Design review of the part built by this model. Coordinates are the model's own, in mm. A direction names the side the tool comes from. Give positions to 0.01 mm unless a question says otherwise; leave off trailing zeros. Loops run counter-clockwise (first coordinate to the right, second up) from the corner with the lowest first, then second, coordinate; pieces in that order, holes last. Notation, with made-up numbers: (40.5, 68) - (82.5, 68) arc R27 cw to (82.5, 89) - close; hole circle Ø8 at (84.5, -14.75). An arc over 180 degrees is marked (long way). One line per item, written item: value. Start each with the question number.
```python
from build123d import *

# Parameters (mm, degrees)
F0_R     = 6.2
F0_R_2   = 5
F1_DEPTH = 10
F0_R_3   = 3.8
F2_DEPTH = 20
F3_SIZE  = 0.5


with BuildPart() as f1:
    # F0 (on Top) → F1 (new body)
    with BuildSketch(Plane.XY):
        Circle(F0_R)
        Circle(F0_R_2, mode=Mode.SUBTRACT)
    extrude(amount=F1_DEPTH)

    # F0 (on Top) → F2 (join)
    with BuildSketch(Plane.XY):
        Circle(F0_R_2)
        Circle(F0_R_3, mode=Mode.SUBTRACT)
    extrude(amount=F2_DEPTH)

    # F3
    f3_edges = [f1.edges().sort_by_distance(p)[0] for p in [
        (-5, 0, 20),
    ]]
    chamfer(f3_edges, length=F3_SIZE)


solid = f1.part
```
(1) To check wall thickness, follow L1, parallel to Y at x = 0, z = 8; L2, parallel to Z at x = -2.5, y = 5; L3, parallel to Y at x = -1.75, z = 3. State the ranges of each line that lie inside material, in increasing order. Write a range as from..to.
(2) Take a section at C-C on z = 2. State the section outline as (x, y) points, and give its area (3 significant figures).
(3) Take a section at D-D on z = 12.5. State the section outline as (x, y) points.
(4) Machinability: for faces 1 (the cylindrical face through (-1.08, -4.88, 14.68)), 2 (the flat face through (-4, -1, 20)), which of the approach directions +Z, -Z, +X, -X, +Y, -Y give a long, thin tool a straight path to every point of the face, cutting with its end or side? Answer none if there is none.
(5) For pin 1 Ø1.5 at (x, y) = (-4.5, 3.5) entering from +Z; pin 2 Ø1.5 at (x, z) = (5, 5) entering from +Y; pin 3 Ø1.5 at (y, z) = (4, 12.5) entering from -X, all flat-tipped, find the tip position at first contact; note any pin that passes through.
(6) Take a section at A-A on y = 0. State the section outline as (x, z) points.
(7) Draft analysis for pull direction X (two halves, no side actions). For faces 3 (the cylindrical face through (2.86, -5.5, 4.93)), 4 (the flat face through (3, 3, 0)), 5 (the cylindrical face through (-3.796, 0.167, 9.86)), state which applies: pulls with the +X half, pulls with the -X half, needs draft (parallel to the pull), parting line crosses it, or undercut.
Here are the results:
1. L1: -6.2..-3.8, 3.8..6.2
1. L2: 0..10
1. L3: -5.95..-3.37, 3.37..5.95
2. outline: circle Ø12.4 at (0, 0); hole circle Ø7.6 at (0, 0)
2. area: 75.4 mm²
3. outline: circle Ø10 at (0, 0); hole circle Ø7.6 at (0, 0)
4. face 1: +Z
4. face 2: +Z, +X, -X, +Y, -Y
5. pin 1: z = 19.55
5. pin 2: y = 4.51
5. pin 3: x = -3.8
6. outline: (-6.2, 0) - (-3.8, 0) - (-3.8, 20) - (-4.5, 20) - (-5, 19.5) - (-5, 10) - (-6.2, 10) - close; (3.8, 0) - (6.2, 0) - (6.2, 10) - (5, 10) - (5, 19.5) - (4.5, 20) - (3.8, 20) - close
7. face 3: parting line crosses it
7. face 4: needs draft
7. face 5: undercut
